Model file for the job. Use its own axes, mm. A direction names the side the tool comes from. Coordinates: 2 decimals unless noted, no trailing zeros. Write each loop counter-clockwise with the first axis right and the second up, starting at its lowest first coordinate (ties: lowest second). Pieces come first, ordered by that corner, then holes.
Q1. Which spindle directions (+Z, -Z, +X, -X, +Y, -Y) get a long thin tool onto all of the face, cutting with end or side? Do faces 1 (the flat face through (0, 1, -19)), 2 (the cylindrical face through (-2.38, 30.39, -10.74)), 3 (the flat face through (6, 9, -20)). Say none if no direction does.
Q2. Band-saw the part on C-C, the plane y = 50.5. Write the cut outline in (x, z), plus the area to 3 significant figures.
Q3. Band-saw the part on A-A, the plane z = 0. Write the cut outline in (x, y).
Q4. Drill centre lines: probe 1 along Z at (x, y) = (15, 0.6); probe 2 along Z at (x, y) = (0, 5). Where is each one in solid material? Low to high.
Q5. Band-saw the part on B-B, the plane x = 2. Write the cut outline in (y, z).
Q6. Band-saw the part on D-D, the plane z = 7.5. Write the cut outline in (x, y), plus the area to 3 significant figures.
Q7. Pull direction X, two halves, no side cores. Call faces 4 (the cylindrical face through (-2.018, 36.171, 15.368)), 5 (the flat face through (5, 13, -15)), 6 (the cylindrical face through (14.84, 0.79, -13.76)): released by +X, released by -X, zero draft, split by the parting line, or undercut.
Q8. Pin check, flat tips, straight feed: P1, Ø3, axis at x = 15, z = -15, coming from the +Y side; P2, Ø6, axis at x = -9.5, z = -7.5, coming from the -Y side; P3, Ø12, axis at x = 9.5, y = 32, coming from the -Z side; P4, Ø3, axis at y = 48, z = 8.5, coming from the -X side. Stop position of each tip, or through.
Autodesk Fusion 360 part; units mm, degrees
sketch "camera_dimensions" plane through (0, 0, 0) normal (0, 1, 0) x (1, 0, 0)
  line L0 (19, -19) -> (-19, -19)
  line L1 (-19, -19) -> (-19, 19)
  line L2 (-19, 19) -> (19, 19)
  line L3 (19, 19) -> (19, -19)
  line L4 (19, -19) -> (-19, 19) construction
  line L5 (-19, -19) -> (19, 19) construction
  circle A0 centre (-15, 15) radius 1.25
  circle A1 centre (15, 15) radius 1.25
  circle A2 centre (-15, -15) radius 1.25
  circle A3 centre (15, -15) radius 1.25
  circle A4 centre (0, 0) radius 18
  circle A5 centre (0, 0) radius 15.5
  circle A6 centre (0, 0) radius 11
  line L6 (-6, 16) -> (6, 16)
  line L7 (6, 16) -> (6, 23)
  line L8 (6, 23) -> (-6, 23)
  line L9 (-6, 23) -> (-6, 16)
  line L10 (0, 30) -> (0, -25) construction
  dimension "d1" = 38
  dimension "d2" = 38
  dimension "d3" = 2.5
  dimension "d4" = 4
  dimension "d5" = 4
  dimension "d6" = 2.5
  dimension "d7" = 2.5
  dimension "d8" = 2.5
  dimension "d9" = 4
  dimension "d10" = 4
  dimension "d11" = 4
  dimension "d12" = 4
  dimension "d13" = 4
  dimension "d14" = 4
  dimension "d15" = 36
  dimension "d16" = 31
  dimension "d17" = 22
  dimension "d18" = 12
extrude "Extrude1" add sketch "camera_dimensions" along normal blind 1.6 contours L0 L1 L2 L3 A4 L7 L9 | L2 A4 L7 L9 | A4 L6 L7 L9 | A4 L6 L7 L9 | A5 | A6
extrude "Extrude2" add sketch "camera_dimensions" along normal blind 11.4 from surface at 1.6 contours A4 L6 L7 L9 | A4 L6 L7 L9 | A5
extrude "Extrude3" add sketch "camera_dimensions" along normal blind 60 contours A5
extrude "Extrude4" add sketch "camera_dimensions" along normal blind 5.2 from surface at 6.6 contours L2 A4 L7 L9 | L2 L7 L8 L9
Answer sheet:
1. face 1: -Z, +X, -X, -Y
1. face 2: +Y
1. face 3: -Z, +X, +Y
2. outline: circle Ø31 at (0, 0); hole circle Ø22 at (0, 0)
2. area: 375 mm2
3. outline: (-19, 0) - (19, 0) - (19, 1.6) - (18, 1.6) - (18, 13) - (15.5, 13) - (15.5, 60) - (11, 60) - (11, 1.6) - (-11, 1.6) - (-11, 60) - (-15.5, 60) - (-15.5, 13) - (-18, 13) - (-18, 1.6) - (-19, 1.6) - close
4. probe 1: z = -19 to -16.25, -13.75 to 13.75, 16.25 to 19
4. probe 2: z = -18 to -11, 11 to 18
5. outline: (0, -19) - (1.6, -19) - (1.6, -17.89) - (6.6, -17.89) - (6.6, -23) - (11.8, -23) - (11.8, -17.89) - (13, -17.89) - (13, -15.37) - (60, -15.37) - (60, -10.82) - (1.6, -10.82) - (1.6, 10.82) - (60, 10.82) - (60, 15.37) - (13, 15.37) - (13, 17.89) - (1.6, 17.89) - (1.6, 19) - (0, 19) - close
6. outline: (-19, 0) - (19, 0) - (19, 1.6) - (16.36, 1.6) - (16.36, 13) - (13.56, 13) - (13.56, 60) - (8.05, 60) - (8.05, 1.6) - (-8.05, 1.6) - (-8.05, 60) - (-13.56, 60) - (-13.56, 13) - (-16.36, 13) - (-16.36, 1.6) - (-19, 1.6) - close
6. area: 769 mm2
7. face 4: split by the parting line
7. face 5: zero draft
7. face 6: undercut
8. P1: stops at y = 1.6
8. P2: stops at y = 0
8. P3: stops at z = -15.1
8. P4: stops at x = -13.83
